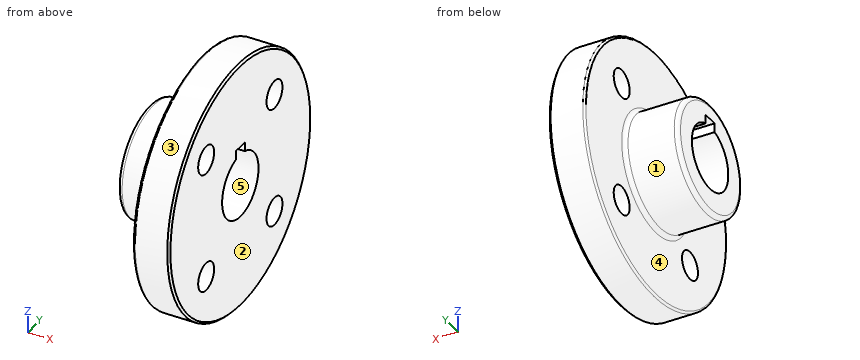
from build123d import *

# Parameters (mm, degrees)
F2_W     = 8
F2_H     = 8
F3_DEPTH = 45.001
F5_D     = 14
F6_R     = 2
F7_R     = 1
F8_SIZE  = 1


with BuildPart() as f1:
    # F0 (on Front) → F1 (revolve)
    with BuildSketch(Plane.XZ):
        Polygon((-45, 16), (0, 16), (0, 62.5), (-18, 62.5), (-18, 28), (-45, 28), align=None)
    revolve(axis=Axis((-18.421089, 0, 0), (1, 0, 0)))

    # F2 (on face) → F3 (cut, through all)
    with BuildSketch(Plane(origin=(-45, 0, 0), x_dir=(0, -1, 0), z_dir=(-1, 0, 0))):
        with Locations((0, 16)):
            Rectangle(F2_W, F2_H)
    extrude(amount=-F3_DEPTH, mode=Mode.SUBTRACT)

    # F5 (through all)
    with Locations(Plane(origin=(-18, 0, 0), x_dir=(0, -1, 0), z_dir=(-1, 0, 0))):
        with Locations((-30.052038, 30.052038), (-30.052038, -30.052038), (30.052038, -30.052038), (30.052038, 30.052038)):
            Hole(F5_D / 2)

    # F6
    f6_edges = [f1.edges().sort_by_distance(p)[0] for p in [
        (-45, 0, -28),
        (-18, 0, -28),
    ]]
    fillet(f6_edges, radius=F6_R)

    # F7
    f7_edges = [f1.edges().sort_by_distance(p)[0] for p in [
        (-18, 0, -62.5),
    ]]
    fillet(f7_edges, radius=F7_R)

    # F8
    f8_edges = [f1.edges().sort_by_distance(p)[0] for p in [
        (0, 0, -62.5),
    ]]
    chamfer(f8_edges, length=F8_SIZE)


solid = f1.part
Work out the finished part from the listing and answer in its coordinate system (mm). Face numbers are marked on the shaded views. A direction names the side the tool comes from. Coordinates: 2 decimals unless noted, no trailing zeros. Write each loop counter-clockwise with the first axis right and the second up, starting at its lowest first coordinate (ties: lowest second). Pieces come first, ordered by that corner, then holes. Notation, with made-up numbers: (85, 76) - (94, 76) arc R11 ccw to (94, 96) - close; hole circle Ø4 at (-21.5, -9.75). An arc over 180 degrees is marked (long way). One line per question, with ' | ' between items.
1) Flat-ended cylindrical pins translate along their axes: P1, Ø1, axis at x = -19.5, z = -14.5, coming from the +Y side; P2, Ø1.5, axis at x = -10, z = -9.5, coming from the -Y side; P3, Ø3.5, axis at x = -22.5, z = 18.5, coming from the -Y side; P4, Ø11, axis at y = 30.05, z = 30.05, coming from the -X side. Find the tip coordinate at first contact, or state that the pin passes through.
Checks:
P1: y = 24.39 | P2: y = -61.88 | P3: y = -22.44 | P4: through
2) The mould has two halves that part along Z. Classify the marked faces 3, 4 and 5: +Z half, -Z half, draft (parallel to the pull), parting line (faces both ways), or undercut.
Checks:
face 3: parting line | face 4: draft | face 5: undercut
3) Find section D-D, the plane x = -15. Determine the outline of the cut face in (y, z), and give its area (3 significant figures).
Checks:
outline: circle Ø125 at (0, 0); hole circle Ø14 at (-30.05, -30.05); hole circle Ø14 at (-30.05, 30.05); hole (-4, 15.49) arc R16 ccw (long way) to (4, 15.49) - (4, 20) - (-4, 20) - close; hole circle Ø14 at (30.05, -30.05); hole circle Ø14 at (30.05, 30.05) | area: 10,800 mm2
4) Find section A-A, the plane y = 0. Determine the outline of the cut face in (x, z).
Checks:
outline: (-45, -26) arc R2 ccw to (-43, -28) - (-20, -28) arc R2 cw to (-18, -30) - (-18, -61.5) arc R1 ccw to (-17, -62.5) - (-1, -62.5) - (0, -61.5) - (0, -16) - (-45, -16) - close; (-45, 20) - (0, 20) - (0, 61.5) - (-1, 62.5) - (-17, 62.5) arc R1 ccw to (-18, 61.5) - (-18, 30) arc R2 cw to (-20, 28) - (-43, 28) arc R2 ccw to (-45, 26) - close
5) Find section C-C, the plane x = -32. Determine the outline of the cut face in (y, z).
Checks:
outline: circle Ø56 at (0, 0); hole (-4, 15.49) arc R16 ccw (long way) to (4, 15.49) - (4, 20) - (-4, 20) - close
6) For the marked faces 1 and 2, determine the directions among +Z, -Z, +X, -X, +Y, -Y from which every point of the face is accessible in a straight line to the end or side of a thin tool.
Checks:
face 1: -X | face 2: +Z, -Z, +X, +Y, -Y
7) Find section B-B, the plane z = 0. Determine the outline of the cut face in (x, y).
Checks:
outline: (-45, -26) arc R2 ccw to (-43, -28) - (-20, -28) arc R2 cw to (-18, -30) - (-18, -61.5) arc R1 ccw to (-17, -62.5) - (-1, -62.5) - (0, -61.5) - (0, -16) - (-45, -16) - close; (-45, 16) - (0, 16) - (0, 61.5) - (-1, 62.5) - (-17, 62.5) arc R1 ccw to (-18, 61.5) - (-18, 30) arc R2 cw to (-20, 28) - (-43, 28) arc R2 ccw to (-45, 26) - close
8) Consider probe 1 along Z at (x, y) = (-11, 0); probe 2 along Z at (x, y) = (-35, 0); probe 3 along X at (y, z) = (-20.5, -41.5). Determine where each line is inside the solid, lowest interval first. Write a range as [from, to].
Checks:
probe 1: [-62.5, -16], [20, 62.5] | probe 2: [-28, -16], [20, 28] | probe 3: [-18, 0]
